```python
from build123d import *

# Parameters (mm, degrees)
SKETCH4_R           = 42.545
BOSS_EXTRUDE2_DEPTH = 0.79375
SKETCH5_R           = 15.875
CUT_EXTRUDE5_DEPTH  = 1.79375
SKETCH9_R           = 3.175
CUT_EXTRUDE12_DEPTH = 1.79375


with BuildPart() as part:
    # Sketch4 → Boss-Extrude2 (new body)
    with BuildSketch(Plane.XY):
        Circle(SKETCH4_R)
    extrude(amount=BOSS_EXTRUDE2_DEPTH)

    # Sketch5 → Cut-Extrude5 (cut, through all)
    with BuildSketch(Plane.XY.offset(0.79375)):
        Circle(SKETCH5_R)
    extrude(amount=-CUT_EXTRUDE5_DEPTH, mode=Mode.SUBTRACT)

    # Sketch9 → Cut-Extrude12 (cut, through all)
    with BuildSketch(Plane.XY.offset(0.79375)):
        with Locations((22.225, 0)):
            Circle(SKETCH9_R)
        with Locations((36.195, 0)):
            Circle(SKETCH9_R)
        with Locations((15.715448212, -15.715448212)):
            Circle(SKETCH9_R)
        with Locations((25.593729945, -25.593729945)):
            Circle(SKETCH9_R)
        with Locations((0, -22.225)):
            Circle(SKETCH9_R)
        with Locations((0, -36.195)):
            Circle(SKETCH9_R)
        with Locations((-15.715448212, -15.715448212)):
            Circle(SKETCH9_R)
        with Locations((-25.593729945, -25.593729945)):
            Circle(SKETCH9_R)
        with Locations((-22.225, 0)):
            Circle(SKETCH9_R)
        with Locations((-36.195, 0)):
            Circle(SKETCH9_R)
        with Locations((-15.715448212, 15.715448212)):
            Circle(SKETCH9_R)
        with Locations((-25.593729945, 25.593729945)):
            Circle(SKETCH9_R)
        with Locations((0, 22.225)):
            Circle(SKETCH9_R)
        with Locations((0, 36.195)):
            Circle(SKETCH9_R)
        with Locations((15.715448212, 15.715448212)):
            Circle(SKETCH9_R)
        with Locations((25.593729945, 25.593729945)):
            Circle(SKETCH9_R)
    extrude(amount=-CUT_EXTRUDE12_DEPTH, mode=Mode.SUBTRACT)


solid = part.part
```
Geometry: final body of the model. Coordinates: model frame, mm. Coordinates: 2 decimals unless noted, no trailing zeros. Order: outer loops, then holes, each group sorted by start corner. A loop starts at its lowest first (then second) coordinate and runs counter-clockwise, first axis right, second up. Notation, with made-up numbers: (76.5, 6) -> (80.5, 6) arc R15 ccw to (80.5, 24) -> close; hole circle Ø8 at (32.25, 36). An arc over 180 degrees is marked (long way). Use CSV: the item, a comma, the result in double quotes.
1) Section A-A on x = 0. Output: boundary loops of the cut face in (y, z) (3 decimals), then the cut area to 3 significant figures.
Findings:
outline,"(-42.545, 0) -> (-39.37, 0) -> (-39.37, 0.794) -> (-42.545, 0.794) -> close; (-33.02, 0) -> (-25.4, 0) -> (-25.4, 0.794) -> (-33.02, 0.794) -> close; (-19.05, 0) -> (-15.875, 0) -> (-15.875, 0.794) -> (-19.05, 0.794) -> close; (15.875, 0) -> (19.05, 0) -> (19.05, 0.794) -> (15.875, 0.794) -> close; (25.4, 0) -> (33.02, 0) -> (33.02, 0.794) -> (25.4, 0.794) -> close; (39.37, 0) -> (42.545, 0) -> (42.545, 0.794) -> (39.37, 0.794) -> close"
area,"22.2 mm^2"
2) Pin query (flat end, axial travel): pin 1 Ø1.5 at (x, y) = (10, 11) entering from -Z. Return the tip coordinate at first contact, or that it passes through.
Findings:
pin 1,"passes through"
3) Line query: line 1 (Y direction, x = -28, z = 0.2); line 2 (X direction, y = 23, z = 0.75); line 3 (Y direction, x = 0, z = 0.45) (3 decimals). Output: solid intervals per line, ascending.
Findings:
line 1,"y = -32.03 to -27.67, -23.52 to 23.52, 27.67 to 32.03"
line 2,"x = -35.79 to -27.42, -23.76 to -3.08, 3.08 to 23.76, 27.42 to 35.79"
line 3,"y = -42.545 to -39.37, -33.02 to -25.4, -19.05 to -15.875, 15.875 to 19.05, 25.4 to 33.02, 39.37 to 42.545"
4) Section D-D on y = 27. Output: boundary loops of the cut face in (x, z), then the cut area to 3 significant figures.
Findings:
outline,"(-32.88, 0) -> (-28.44, 0) -> (-28.44, 0.79) -> (-32.88, 0.79) -> close; (-22.75, 0) -> (22.75, 0) -> (22.75, 0.79) -> (-22.75, 0.79) -> close; (28.44, 0) -> (32.88, 0) -> (32.88, 0.79) -> (28.44, 0.79) -> close"
area,"43.2 mm^2"
5) Section C-C on z = 0.3. State how many separate pieces and enclosed holes the cut face has, then the cut area to 3 significant figures.
Findings:
separate pieces,"1"
enclosed holes,"17"
area,"4,390 mm^2"
6) Mould query, pull axis Y, two halves, no side actions, for faces 1 (the cylindrical face through (-33.76, -25.89, 0.39)), 2 (the flat face through (-1, -18, 0.794)), 3 (the cylindrical face through (-0.413, 39.343, 0.402)). Classes: +Y half, -Y half, draft (parallel to the pull), parting line (faces both ways), or undercut.
Findings:
face 1,"parting line"
face 2,"draft"
face 3,"undercut"
